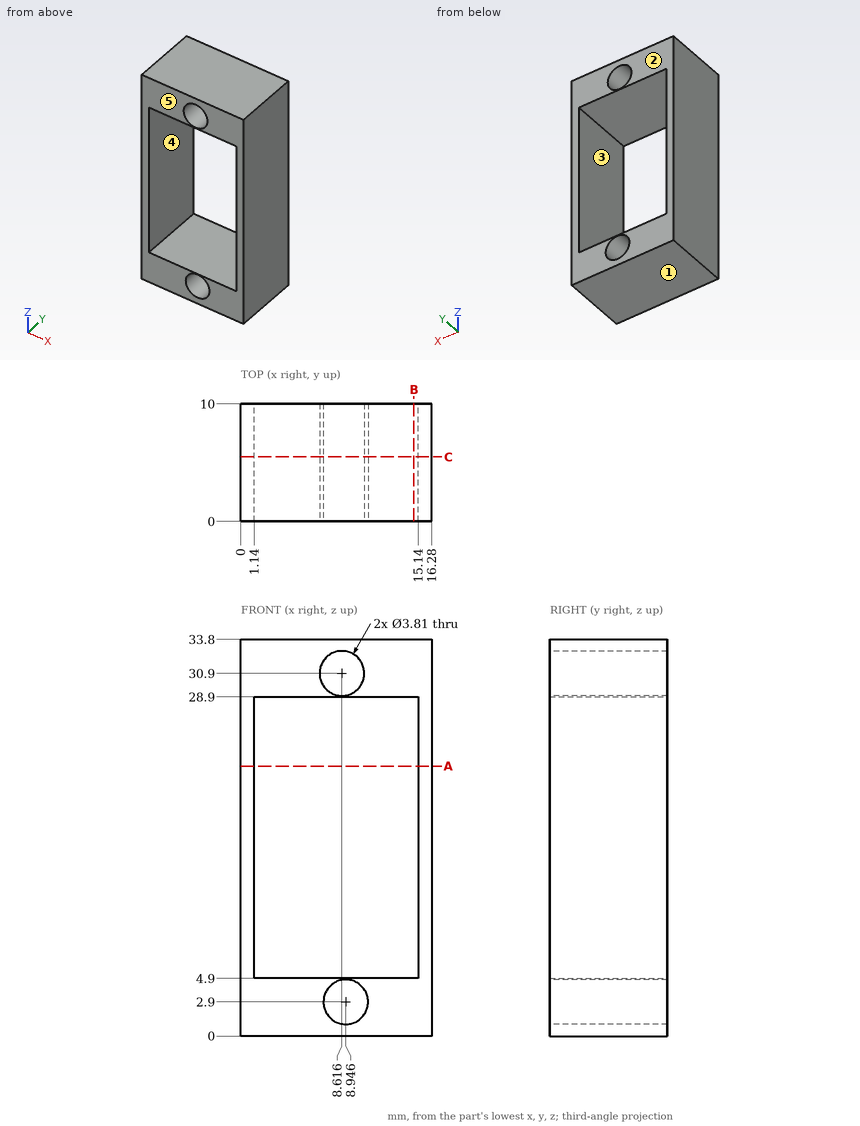
Input: dimensioned drawing with shaded views. Units: mm. Origin: part minimum x, y, z. A direction names the side the tool comes from. Coordinates: 2 decimals unless noted, no trailing zeros. Order: outer loops, then holes, each group sorted by start corner. A loop starts at its lowest first (then second) coordinate and runs counter-clockwise, first axis right, second up. Notation, with made-up numbers: (89, 3) -> (100, 3) arc R27 ccw to (100, 41) -> close; hole circle Ø7 at (-39, -39). An arc over 180 degrees is marked (long way). Use CSV: the item, a comma, the result in double quotes.
1) Access query for the marked faces 4 and 5. Directions: +Z, -Z, +X, -X, +Y, -Y. A direction counts if a zero-diameter tool reaches every point of the face in a straight line with its end or side. Return the directions, or none.
Findings:
face 4,"+Y, -Y"
face 5,"+Z, -Z, +X, -X, -Y"
2) Mould query, pull axis Z, two halves, no side actions, for the marked faces 1, 2 and 3. Classes: +Z half, -Z half, draft (parallel to the pull), parting line (faces both ways), or undercut.
Findings:
face 1,"-Z half"
face 2,"draft"
face 3,"undercut"
3) Section C-C on y = 5.5. Output: boundary loops of the cut face in (x, z) (3 decimals).
Findings:
outline,"(0, 0) -> (16.28, 0) -> (16.28, 33.8) -> (0, 33.8) -> close; hole (1.14, 4.9) -> (15.14, 4.9) -> (15.14, 28.9) -> (1.14, 28.9) -> close; hole circle Ø3.81 at (8.616, 30.9); hole circle Ø3.81 at (8.946, 2.9)"
4) Section B-B on x = 14.75. Output: boundary loops of the cut face in (y, z).
Findings:
outline,"(0, 0) -> (10, 0) -> (10, 4.9) -> (0, 4.9) -> close; (0, 28.9) -> (10, 28.9) -> (10, 33.8) -> (0, 33.8) -> close"
5) Pin query (flat end, axial travel): pin 1 Ø3.5 at (x, z) = (8.95, 2.9) entering from -Y. Return the tip coordinate at first contact, or that it passes through.
Findings:
pin 1,"passes through"
6) Section A-A on z = 23. Output: boundary loops of the cut face in (x, y).
Findings:
outline,"(0, 0) -> (1.14, 0) -> (1.14, 10) -> (0, 10) -> close; (15.14, 0) -> (16.28, 0) -> (16.28, 10) -> (15.14, 10) -> close"
7) Line query: line 1 (X direction, y = 6, z = 30.9); line 2 (X direction, y = 9.25, z = 15); line 3 (Z direction, x = 4, y = 8.5). Output: solid intervals per line, ascending.
Findings:
line 1,"x = 0 to 6.71, 10.52 to 16.28"
line 2,"x = 0 to 1.14, 15.14 to 16.28"
line 3,"z = 0 to 4.9, 28.9 to 33.8"
